Design review of the part built by this model. Coordinates are the model's own, in mm. Face numbers are marked on the shaded views. A direction names the side the tool comes from. Coordinates: 2 decimals unless noted, no trailing zeros. Write each loop counter-clockwise with the first axis right and the second up, starting at its lowest first coordinate (ties: lowest second). Pieces come first, ordered by that corner, then holes. Notation, with made-up numbers: (68.25, -10.5) - (96.25, -10.5) arc R31 ccw to (96.25, 27.5) - close; hole circle Ø4 at (73.25, -2). An arc over 180 degrees is marked (long way). Use a Markdown table: item, result.
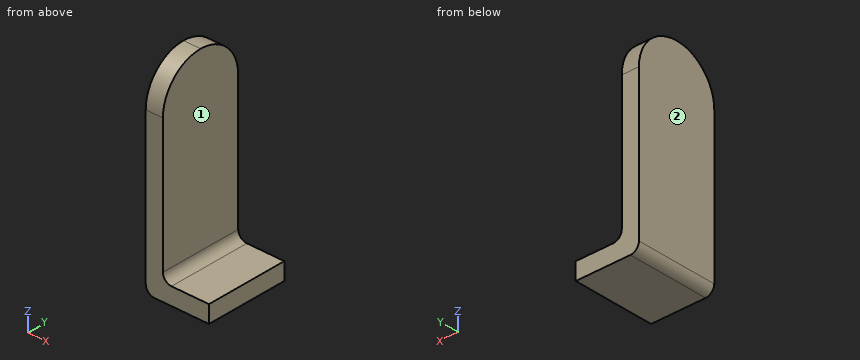
from build123d import *

# Parameters (mm, degrees)
F1_DEPTH = 15.24
F2_R     = 1.5875
F4_DEPTH = 3.175


with BuildPart() as f1:
    # F0 (on Front) → F1 (new body)
    with BuildSketch(Plane.XZ):
        Polygon((3.175, 37.084), (0, 37.084), (0, 0), (11.684, 0), (11.684, 3.175), (3.175, 3.175), align=None)
    extrude(amount=-F1_DEPTH)

    # F2
    f2_edges = [f1.edges().sort_by_distance(p)[0] for p in [
        (3.175, 7.62, 3.175),
        (0, 7.62, 0),
    ]]
    fillet(f2_edges, radius=F2_R)

    # F3 (on face) → F4 (cut, through all)
    with BuildSketch(Plane(origin=(0, 0, 0), x_dir=(0, -1, 0), z_dir=(-1, 0, 0))):
        with BuildLine():
            ThreePointArc((-15.24, 29.464), (-13.0081536726, 34.8521536726), (-7.62, 37.084))
            Line((-7.62, 37.084), (-15.24, 37.084))
            Line((-15.24, 37.084), (-15.24, 29.464))
        make_face()
        with BuildLine():
            ThreePointArc((-7.62, 37.084), (-2.2318463274, 34.8521536726), (0, 29.464))
            Line((0, 29.464), (0, 37.084))
            Line((0, 37.084), (-7.62, 37.084))
        make_face()
    extrude(amount=-F4_DEPTH, mode=Mode.SUBTRACT)


solid = f1.part
(1) Take a section at B-B on y = 13. Write out the cut boundary in (x, z) (1 decimal).
Determined:
| item | result |
|---|---|
| outline | (0, 1.6) arc R1.6 ccw to (1.6, 0) - (11.7, 0) - (11.7, 3.2) - (4.8, 3.2) arc R1.6 cw to (3.2, 4.8) - (3.2, 34.9) - (0, 34.9) - close |
(2) For pin 1 (5 mm diameter, centred on x = 7.5, z = 10, fed in from +Y); pin 2 (3 mm diameter, centred on x = 3.5, z = 13, fed in from -Y); pin 3 (2 mm diameter, centred on y = 3, z = 8, fed in from +X) (3 decimals); pin 4 (3.5 mm diameter, centred on x = 7.5, y = 11, fed in from +Z) (3 decimals), all flat-tipped, find the tip position at first contact; note any pin that passes through.
Determined:
| item | result |
|---|---|
| pin 1 | through |
| pin 2 | y = 0 |
| pin 3 | x = 3.175 |
| pin 4 | z = 3.175 |
(3) Take a section at D-D on y = 6.75. Write out the cut boundary in (x, z) (1 decimal).
Determined:
| item | result |
|---|---|
| outline | (0, 1.6) arc R1.6 ccw to (1.6, 0) - (11.7, 0) - (11.7, 3.2) - (4.8, 3.2) arc R1.6 cw to (3.2, 4.8) - (3.2, 37) - (0, 37) - close |
(4) For L1, parallel to X at y = 8.5, z = 28 (3 decimals); L2, parallel to Z at x = 3.5, y = 6.25, list the stretches that pass through material, from the lowest coordinate up. Write a range as from..to.
Determined:
| item | result |
|---|---|
| L1 | 0..3.175 |
| L2 | 0..3.8 |
(5) Take a section at C-C on z = 22. Write out the cut boundary in (x, y) (3 decimals).
Determined:
| item | result |
|---|---|
| outline | (0, 0) - (3.175, 0) - (3.175, 15.24) - (0, 15.24) - close |
(6) Take a section at A-A on x = 2.5. Write out the cut boundary in (y, z).
Determined:
| item | result |
|---|---|
| outline | (0, 0) - (15.24, 0) - (15.24, 29.46) arc R7.62 ccw to (0, 29.46) - close |
(7) Machinability: for the marked faces 1 and 2, which of the approach directions +Z, -Z, +X, -X, +Y, -Y give a long, thin tool a straight path to every point of the face, cutting with its end or side? Answer none if there is none.
Determined:
| item | result |
|---|---|
| face 1 | +Z, +X, +Y, -Y |
| face 2 | +Z, -Z, -X, +Y, -Y |
